Autodesk Inventor part; units mm, degrees
ref_plane "YZ Plane" through (0, 0, 0) normal (1, 0, 0) x (0, 1, 0)
ref_plane "XZ Plane" through (0, 0, 0) normal (0, 1, 0) x (-1, 0, 0)
ref_plane "XY Plane" through (0, 0, 0) normal (0, 0, 1) x (1, 0, 0)
sketch "Sketch1" plane through (0, 0, 0) normal (0, 1, 0) x (-1, 0, 0)
  line L0 (-15, -15) -> (15, -15)
  line L1 (15, -15) -> (15, 15)
  line L2 (15, 15) -> (-15, 15)
  line L3 (-15, 15) -> (-15, -15)
  line L4 (-15, -15) -> (15, 15) construction
  line L5 (15, -15) -> (-15, 15) construction
  line L6 (-2.45, -12.65) -> (2.45, -12.65) construction
  line L7 (2.45, -12.65) -> (2.45, 12.65) construction
  line L8 (2.45, 12.65) -> (-2.45, 12.65) construction
  line L9 (-2.45, 12.65) -> (-2.45, -12.65) construction
  line L10 (-2.45, -12.65) -> (2.45, 12.65) construction
  line L11 (2.45, -12.65) -> (-2.45, 12.65) construction
  line L12 (-12.65, -2.45) -> (12.65, -2.45) construction
  line L13 (12.65, -2.45) -> (12.65, 2.45) construction
  line L14 (12.65, 2.45) -> (-12.65, 2.45) construction
  line L15 (-12.65, 2.45) -> (-12.65, -2.45) construction
  line L16 (-12.65, -2.45) -> (12.65, 2.45) construction
  line L17 (12.65, -2.45) -> (-12.65, 2.45) construction
  line L18 (-12.85, -2.65) -> (12.85, -2.65)
  line L19 (12.85, -2.65) -> (12.85, 2.65)
  line L20 (12.85, 2.65) -> (-12.85, 2.65)
  line L21 (-12.85, 2.65) -> (-12.85, -2.65)
  line L22 (-12.85, -2.65) -> (12.85, 2.65) construction
  line L23 (12.85, -2.65) -> (-12.85, 2.65) construction
  line L24 (-2.65, -12.85) -> (2.65, -12.85)
  line L25 (2.65, -12.85) -> (2.65, 12.85)
  line L26 (2.65, 12.85) -> (-2.65, 12.85)
  line L27 (-2.65, 12.85) -> (-2.65, -12.85)
  line L28 (-2.65, -12.85) -> (2.65, 12.85) construction
  line L29 (2.65, -12.85) -> (-2.65, 12.85) construction
  point P0 (0, 0)
  point P1 (0, 0)
  dimension "d0" = 30
  dimension "d1" = 4.9
  dimension "d2" = 10.2
  dimension "d3" = 0.2
  dimension "d4" = 0.2
extrude "Extrusion1" add sketch "Sketch1" along normal blind 1.9
sketch "Sketch2" plane through (0, 1.9, 0) normal (0, 1, 0) x (1, 0, 0)
  line L0 (15, 15) -> (-15, 15)
  line L1 (-15, 15) -> (-15, -15)
  line L2 (-15, -15) -> (15, -15)
  line L3 (15, -15) -> (15, 15)
  circle A0 centre (0, 0) radius 1.5
  dimension "d7" = 3
extrude "Extrusion2" add sketch "Sketch2" along normal blind 2
sketch "Sketch3" plane through (0, 3.9, 0) normal (0, 1, 0) x (1, 0, 0)
  circle A0 centre (0, 0) radius 1.5
  line L0 (15, 15) -> (-15, 15)
  line L1 (-15, 15) -> (-15, -15)
  line L2 (-15, -15) -> (15, -15)
  line L3 (15, -15) -> (15, 15)
  circle A1 centre (0, 0) radius 2.75
  dimension "d10" = 5.5
extrude "Extrusion3" add sketch "Sketch3" along normal blind 0.5 contours L3 L2 L1 L0
chamfer "Chamfer1" distance 2 angle 45 1 edges at (-2.65, 0.95, -2.65)
fillet "Fillet1" radius 2.45 1 edges at (-12.85, 0.95, -2.65)
fillet "Fillet2" radius 2.45 1 edges at (-2.65, 0.95, -12.85)
chamfer "Chamfer2" distance 2 angle 45 1 edges at (2.65, 0.95, -2.65)
chamfer "Chamfer3" distance 2 angle 45 1 edges at (2.65, 0.95, 2.65)
fillet "Fillet3" radius 2.45 1 edges at (12.85, 0.95, -2.65)
fillet "Fillet4" radius 2.45 1 edges at (2.65, 0.95, -12.85)
fillet "Fillet5" radius 2.45 1 edges at (12.85, 0.95, 2.65)
fillet "Fillet6" radius 2.45 1 edges at (2.65, 0.95, 12.85)
chamfer "Chamfer4" distance 2 angle 45 1 edges at (-2.65, 0.95, 2.65)
fillet "Fillet7" radius 2.45 2 edges at (-2.65, 0.95, 12.85) (-12.85, 0.95, 2.65)
sketch "Sketch4" plane through (0, 0, 0) normal (0, -1, 0) x (1, 0, 0)
  line L0 (15, -15) -> (-15, -15)
  line L1 (-10.4, 2.65) -> (-4.65, 2.65)
  line L2 (-15, -15) -> (-10, -76.15)
  line L3 (-10, -76.15) -> (10, -76.15)
  line L4 (10, -76.15) -> (15, -15)
  line L5 (0, 0) -> (0, -92.3376) construction
  arc A0 (-10, -76.15) -> (10, -76.15) centre (0, -76.15) ccw
  dimension "d32" = 76.15
  dimension "d33" = 20
extrude "Extrusion4" add sketch "Sketch4" against normal up to surface (4.4 mm away)
sketch "Sketch5" plane through (0, 0, 0) normal (0, -1, 0) x (1, 0, 0)
  line L0 (-5.7, -48.25) -> (5.7, -48.25) construction
  line L1 (5.7, -48.25) -> (5.7, -71.75) construction
  line L2 (5.7, -71.75) -> (-5.7, -71.75) construction
  line L3 (-5.7, -71.75) -> (-5.7, -48.25) construction
  line L4 (0, 0) -> (0, -72.1654) construction
  line L5 (-5.7, -48.25) -> (-5.7, -43.85) construction
  line L6 (-5.7, -43.85) -> (5.7, -43.85) construction
  line L7 (5.7, -43.85) -> (5.7, -48.25) construction
  line L8 (5.7, -71.75) -> (5.7, -76.15) construction
  line L9 (5.7, -76.15) -> (-5.7, -76.15) construction
  line L10 (-5.7, -76.15) -> (-5.7, -71.75) construction
  circle A0 centre (-2.7, -45.85) radius 1.3
  circle A1 centre (2.7, -45.85) radius 1.3
  line L11 (-17.4512, -60) -> (18.2205, -60) construction
  circle A2 centre (-2.7, -74.15) radius 1.3
  circle A3 centre (2.7, -74.15) radius 1.3
  line L12 (-6.2, -47.75) -> (6.2, -47.75)
  line L13 (6.2, -47.75) -> (6.2, -72.25)
  line L14 (6.2, -72.25) -> (-6.2, -72.25)
  line L15 (-6.2, -72.25) -> (-6.2, -47.75)
  dimension "d36" = 11.4
  dimension "d37" = 23.5
  dimension "d38" = 3
  dimension "d39" = 2.4
  dimension "d40" = 4.4
  dimension "d41" = 0.5
  dimension "d42" = 0.5
  dimension "d43" = 60
  dimension "d44" = 2.6
extrude "Extrusion5" cut sketch "Sketch5" against normal through all
sketch "Sketch6" plane through (0, 0, 0) normal (0, -1, 0) x (1, 0, 0)
  arc A0 (-10, -76.15) -> (10, -76.15) centre (0, -76.15) ccw
  line L0 (-5.7, -48.25) -> (5.7, -48.25) construction
  line L1 (5.7, -48.25) -> (5.7, -71.75) construction
  line L2 (5.7, -71.75) -> (-5.7, -71.75) construction
  line L3 (-5.7, -71.75) -> (-5.7, -48.25) construction
  line L4 (0, 0) -> (0, -72.5327) construction
  line L5 (-5.7, -48.25) -> (-5.7, -43.85) construction
  line L6 (-5.7, -43.85) -> (5.7, -43.85) construction
  line L7 (5.7, -43.85) -> (5.7, -48.25) construction
  line L8 (5.7, -71.75) -> (5.7, -76.15) construction
  line L9 (5.7, -76.15) -> (-5.7, -76.15) construction
  line L10 (-5.7, -76.15) -> (-5.7, -71.75) construction
  line L11 (-0.5684, -60) -> (35.1033, -60) construction
  line L12 (-6.2, -43.35) -> (6.2, -43.35)
  line L13 (6.2, -43.35) -> (6.2, -76.65)
  line L14 (6.2, -76.65) -> (-6.2, -76.65)
  line L15 (-6.2, -76.65) -> (-6.2, -43.35)
  dimension "d64" = 11.4
  dimension "d65" = 23.5
  dimension "d68" = 4.4
  dimension "d70" = 0.5
  dimension "d71" = 60
  dimension "d81" = 0.5
extrude "Extrusion6" cut sketch "Sketch6" against normal blind 1.4
equation "\"d0\" = FrontUpperLegShoulderWidth"
equation "\"d1\" = ServoArmWidth"
equation "\"d2\" = ServoArmLength"
equation "\"d3\" = ServoArmSpacing"
equation "\"d4\" = ServoArmSpacing"
equation "\"d5\" = ServoArmThickness"
equation "\"d7\" = ServoArmHoleRequired"
equation "\"d8\" = MinimalThickness"
equation "\"d10\" = ServoArmHeadScrewTrace"
equation "\"d11\" = ServoArmHeadScrewThickness"
equation "\"d13\" = ServoArmInternFillet"
equation "\"d16\" = ServoArmExternFillet"
equation "\"d17\" = ServoArmExternFillet"
equation "\"d18\" = ServoArmInternFillet"
equation "\"d21\" = ServoArmInternFillet"
equation "\"d24\" = ServoArmExternFillet"
equation "\"d25\" = ServoArmExternFillet"
equation "\"d26\" = ServoArmExternFillet"
equation "\"d27\" = ServoArmExternFillet"
equation "\"d28\" = ServoArmInternFillet"
equation "\"d31\" = ServoArmExternFillet"
equation "\"d32\" = 0.5 * ServoCoreLength + FrontUpperLegLength + ServoFixationLength"
equation "\"d33\" = FrontUpperLegKneeWidth"
equation "\"d36\" = ServoCoreWidth"
equation "\"d37\" = ServoCoreLength"
equation "\"d38\" = ServoEdgeToFixation"
equation "\"d39\" = ServoCoreToFixation"
equation "\"d40\" = ServoFixationLength"
equation "\"d41\" = ServoTraceSpacing"
equation "\"d42\" = ServoTraceSpacing"
equation "\"d43\" = FrontUpperLegLength"
equation "\"d44\" = ServoScrewDiameterRequired"
equation "\"d64\" = ServoCoreWidth"
equation "\"d65\" = ServoCoreLength"
equation "\"d68\" = ServoFixationLength"
equation "\"d70\" = ServoTraceSpacing"
equation "\"d71\" = FrontUpperLegLength"
equation "\"d81\" = ServoTraceSpacing"
equation "\"d92\" = ServoArmThickness + ServoArmHeadScrewThickness + MinimalThickness - LegServoThickness"
equation "\"FrontUpperLegLength\" = 60"
equation "\"FrontUpperLegKneeWidth\" = 20"
equation "\"ServoTraceSpacing\" = 0.5"
equation "\"FrontUpperLegShoulderWidth\" = 30"
equation "\"LegServoThickness\" = 3"
properties part number "BackUpperLeg"
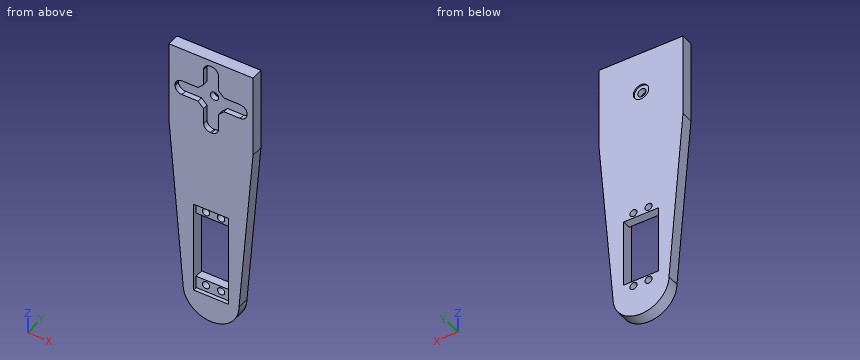
The listing builds one solid part. Answer for the finished solid, in the listing's coordinates (mm). Round coordinates to 2 decimals unless told otherwise and drop trailing zeros. Order: outer loops, then holes, each group sorted by start corner. A loop starts at its lowest first (then second) coordinate and runs counter-clockwise, first axis right, second up. Notation, with made-up numbers: M 50.25,67.5 L 94.25,67.5 A25 ccw 94.25,89.5 Z; hole C 14.5,-1.5 d5. An arc over 180 degrees is marked long. Answer in a Markdown table with one row per item. Add a question column.
1) The part is cut by section A-A on z = -8. Determine the outline of the cut face in (x, y), plus the area to 3 significant figures.
2) Consider line 1 along Z through (x, y) = (0, 4.25); line 2 along X through (y, z) = (4.25, 0); line 3 along Z through (x, y) = (4, 0.9). Determine where each line is inside the solid, lowest interval first. Write a range as from..to.
3) The part is cut by section D-D on z = -30. Determine the outline of the cut face in (x, y), plus the area to 3 significant figures.
4) The part is cut by section C-C on z = -65.5. Determine the outline of the cut face in (x, y), plus the area to 3 significant figures.
5) Flat-ended cylindrical pins translate along their axes: pin 1 Ø3.5 at (x, z) = (2, -45.5) entering from -Y; pin 2 Ø4.5 at (x, z) = (0, 0) entering from -Y. Find the tip coordinate at first contact, or state that the pin passes through.
6) The part is cut by section B-B on x = 8. Determine the outline of the cut face in (y, z), plus the area to 3 significant figures.
Findings below:
| question | item | result |
|---|---|---|
| 1 | outline | M -15,0 L -2.65,0 L -2.65,1.9 L 2.65,1.9 L 2.65,0 L 15,0 L 15,4.4 L -15,4.4 Z |
| 1 | area | 122 mm² |
| 2 | line 1 | z = -86.15..-72.25, -47.75..-2.75, 2.75..15 |
| 2 | line 2 | x = -15..-2.75, 2.75..15 |
| 2 | line 3 | z = -85.32..-76.65, -43.35..-3.3, 3.3..15 |
| 3 | outline | M -13.77,0 L 13.77,0 L 13.77,4.4 L -13.77,4.4 Z |
| 3 | area | 121 mm² |
| 4 | outline | M -10.87,0 L -6.2,0 L -6.2,4.4 L -10.87,4.4 Z; M 6.2,0 L 10.87,0 L 10.87,4.4 L 6.2,4.4 Z |
| 4 | area | 41.1 mm² |
| 5 | pin 1 | stops at y = 1.4 |
| 5 | pin 2 | stops at y = 1.9 |
| 6 | outline | M 0,-82.15 L 4.4,-82.15 L 4.4,15 L 0,15 L 0,2.65 L 1.9,2.65 L 1.9,-2.65 L 0,-2.65 Z |
| 6 | area | 417 mm² |
